Part model, mm, in its own coordinate system. A direction names the side the tool comes from. Round coordinates to 2 decimals unless told otherwise and drop trailing zeros. Order: outer loops, then holes, each group sorted by start corner. A loop starts at its lowest first (then second) coordinate and runs counter-clockwise, first axis right, second up. Notation, with made-up numbers: (-16, 84) -> (4, 84) arc R5 ccw to (4, 93) -> close; hole circle Ø2 at (51.5, -22). An arc over 180 degrees is marked (long way). Answer as a JSON object with one key per item and string values. Group by question number.
```python
from build123d import *

# Parameters (mm, degrees)
CUT_EXTRUDE1_DEPTH      = 10
CUT_EXTRUDE1_DEPTH_BACK = 10
SKETCH7_W               = 161.67088451347962
SKETCH7_H               = 99.40268669666085
SKETCH8_W               = 4.999999999999993
SKETCH8_H               = 94
CUT_EXTRUDE2_DEPTH      = 35
SKETCH9_R               = 7.5
SKETCH9_R_2             = 4.000000000000013
SKETCH9_R_3             = 4.000000000000005
CUT_EXTRUDE3_DEPTH      = 357.06460088023357
SKETCH10_R              = 4.000000000000005
CUT_EXTRUDE4_DEPTH      = 386.9080201291493
SKETCH11_W              = 141.9999999999999
SKETCH11_H              = 16
BOSS_EXTRUDE1_DEPTH     = 330
FILLET2_R               = 5
FILLET3_R               = 5
FILLET4_R               = 5
FILLET5_R               = 5
FILLET6_R               = 5
CUT_EXTRUDE5_DEPTH      = 389.0992141192763


with BuildPart() as part:
    # Sweep2: sweep along a path in Sketch4
    with BuildLine(Plane.XY) as sweep2_path:
        Line((-65, 350), (-64.99999999999994, 10.000000000000007))
        ThreePointArc((-64.99999999999994, 10.000000000000007), (-62.07106781186544, 2.928932188134527), (-54.99999999999996, 0))
        Line((-54.99999999999996, 0), (54.99999999999999, 0))
        ThreePointArc((54.99999999999999, 0), (62.071067811865476, 2.9289321881345227), (65, 10))
        Line((65, 10), (65, 350))
        Line((65, 350), (-65, 350))
    # Sketch6 → Sweep2 (sweep)
    with BuildSketch(Plane(origin=(0, 0, 0), x_dir=(0, 0, -1), z_dir=(1, 0, 0))):
        Polygon((45.00000000000006, 355.99999999999994), (-44.999999999999936, 355.99999999999994), (-44.999999999999936, 343.99999999999994), (45.000000000000064, 344), align=None)
    sweep(path=sweep2_path.line, transition=Transition.RIGHT)

    # Sketch7 → Cut-Extrude1 (cut, two sides: drawn at the far end of the back side and taken through both)
    with BuildSketch(Plane(origin=(0, 0, 0), x_dir=(1, 0, 0), z_dir=(0, 1, 0)).offset(-CUT_EXTRUDE1_DEPTH_BACK)):
        Rectangle(SKETCH7_W, SKETCH7_H)
    extrude(amount=CUT_EXTRUDE1_DEPTH + CUT_EXTRUDE1_DEPTH_BACK, mode=Mode.SUBTRACT)

    # Sketch8 → Cut-Extrude2 (cut)
    with BuildSketch(Plane(origin=(0, 0, 0), x_dir=(1, 0, 0), z_dir=(0, 1, 0))):
        with Locations((-65.5, 0.24224418482823395)):
            Rectangle(SKETCH8_W, SKETCH8_H)
        with Locations((65.5, 0.24224418482823395)):
            Rectangle(SKETCH8_W, SKETCH8_H)
    extrude(amount=CUT_EXTRUDE2_DEPTH, mode=Mode.SUBTRACT)

    # Sketch9 → Cut-Extrude3 (cut, through all)
    with BuildSketch(Plane(origin=(0, 355.99999999999994, 0), x_dir=(1, 0, 0), z_dir=(0, 1, 0))):
        with Locations(Location((0, 0, 0), (0, 0, 270))):
            Circle(SKETCH9_R)
        with Locations(Location((-42, 31.999999999999993, 0), (0, 0, 270))):
            Circle(SKETCH9_R_2)
        with Locations(Location((-42, -32.00000000000001, 0), (0, 0, 270))):
            Circle(SKETCH9_R_3)
        with Locations(Location((42, -31.999999999999954, 0), (0, 0, 90))):
            Circle(SKETCH9_R_3)
        with Locations(Location((42, 32, 0), (0, 0, 90))):
            Circle(SKETCH9_R_2)
    extrude(amount=-CUT_EXTRUDE3_DEPTH, mode=Mode.SUBTRACT)

    # Sketch10 → Cut-Extrude4 (cut, through all)
    with BuildSketch(Plane(origin=(70.99999999999996, 0, 0), x_dir=(0, 0, -1), z_dir=(1, 0, 0))):
        with Locations((-37.999999999999936, 17.000000000000014)):
            Circle(SKETCH10_R)
    extrude(amount=-CUT_EXTRUDE4_DEPTH, mode=Mode.SUBTRACT)

    # Sketch11 → Boss-Extrude1 (add)
    with BuildSketch(Plane(origin=(0, 355.99999999999994, 0), x_dir=(1, 0, 0), z_dir=(0, 1, 0))):
        with Locations((0, -52.999999999999936)):
            Rectangle(SKETCH11_W, SKETCH11_H)
    extrude(amount=-BOSS_EXTRUDE1_DEPTH)

    # Fillet2
    fillet2_edges = [part.edges().sort_by_distance(p)[0] for p in [
        (59.00000000000001, 177, -45.000000000000064),
    ]]
    fillet(fillet2_edges, radius=FILLET2_R)

    # Fillet3
    fillet3_edges = [part.edges().sort_by_distance(p)[0] for p in [
        (70.99999999999994, 182.99999999999997, -45.00000000000005),
    ]]
    fillet(fillet3_edges, radius=FILLET3_R)

    # Fillet4
    fillet4_edges = [part.edges().sort_by_distance(p)[0] for p in [
        (-59.00000000000001, 177, -45.000000000000064),
    ]]
    fillet(fillet4_edges, radius=FILLET4_R)

    # Fillet5
    fillet5_edges = [part.edges().sort_by_distance(p)[0] for p in [
        (-70.99999999999994, 182.99999999999997, -45.00000000000005),
    ]]
    fillet(fillet5_edges, radius=FILLET5_R)

    # Fillet6
    fillet6_edges = [part.edges().sort_by_distance(p)[0] for p in [
        (70.99999999999994, 355.99999999999994, 10.499999999999893),
        (69.53553390593268, 355.9999999999999, -43.535533905932894),
        (0, 355.99999999999994, -45.00000000000005),
        (0, 355.99999999999994, -45.00000000000005),
        (-69.53553390593268, 355.99999999999994, -43.535533905932795),
        (-70.99999999999994, 355.99999999999994, 10.499999999999936),
        (0, 355.99999999999994, 60.999999999999936),
        (-70.99999999999994, 190.99999999999994, 60.999999999999936),
        (70.99999999999994, 190.99999999999994, 60.999999999999936),
    ]]
    fillet(fillet6_edges, radius=FILLET6_R)

    # Sketch12 → Cut-Extrude5 (cut, through all)
    with BuildSketch(Plane.ZY.offset(70.9999999999999)):
        with BuildLine():
            Line((-19.99811023879916, 9.999999999999995), (-79.77303285275339, 10.000000000000018))
            Line((-79.77303285275339, 10.000000000000018), (-79.77303285275339, 406.4421165391139))
            Line((-79.77303285275339, 406.4421165391139), (-12.883579031367276, 360.2403098799698))
            ThreePointArc((-12.883579031367276, 360.2403098799698), (-23.51999666611846, 185.26395577223084), (-19.99811023879916, 9.999999999999995))
        make_face()
    extrude(amount=-CUT_EXTRUDE5_DEPTH, mode=Mode.SUBTRACT)


solid = part.part
```
Q1. Wall check: line 1 (X direction, y = 350, z = 32); line 2 (X direction, y = 28, z = -2); line 3 (X direction, y = 148, z = -1.5). Give the ranges that are in metal, low to high. Write a range as [from, to].
Q2. Band-saw the part on C-C (y = 17). Count the separate pieces of the cut face and the enclosed holes in it, plus the area to 3 significant figures.
Q3. Which spindle directions (+Z, -Z, +X, -X, +Y, -Y) get a long thin tool onto all of the face, cutting with end or side? Do faces 4 (the flat face through (-68, 22, 12)), 5 (the cylindrical face through (62.78, 222.418, -22.447)). Say none if no direction does.
Q4. Band-saw the part on D-D (x = 20). List the corners of the cut face in (y, z).
Q5. Band-saw the part on A-A (z = 0). List the corners of the cut face in (x, y).
Q6. Drop flat-ended pins along their axis: pin 1 Ø2 at (x, y) = (-15, 68.5) entering from -Z; pin 2 Ø5.5 at (x, z) = (64.5, 25) entering from -Y; pin 3 Ø18 at (x, z) = (-10.5, 13.5) entering from -Y; pin 4 Ø13 at (x, z) = (-8, 54.5) entering from -Y. Give the stop position or say it passes through.
Q7. Two-plate mould, pull along Z, no slides. Class faces 1 (the flat face through (-1, 191, 61)), 2 (the flat face through (-1, 344, 16)), 3 (the cylindrical face through (-69.48, 19.7, 40.95)): +Z half, -Z half, draft (parallel to the pull), parting line (faces both ways), or undercut.
Q8. Band-saw the part on B-B (x = 42). List the corners of the cut face in (y, z), plus the area to 3 significant figures.
Completed:
{
 "1": {"line 1": "[-71, -46], [-38, 38], [46, 71]", "line 2": "[-71, -68], [-63, -59], [59, 63], [68, 71]", "line 3": "[-71, -59], [59, 71]"},
 "2": {"separate pieces": "8", "enclosed holes": "0", "area": "804 mm2"},
 "3": {"face 4": "-Z, -Y", "face 5": "-Z, +X, -X"},
 "4": {"outline": "(26, 45) -> (344, 45) -> (344, -14.47) arc R2170 ccw to (356, -13.31) -> (356, 56) arc R5 ccw to (351, 61) -> (26, 61) -> close"},
 "5": {"outline": "(-71, 10) -> (-68, 10) -> (-68, 35) -> (-63, 35) -> (-63, 10) -> (-59, 10) -> (-59, 344) -> (-7.5, 344) -> (-7.5, 356) -> (-66, 356) arc R5 ccw to (-71, 351) -> close; (7.5, 344) -> (59, 344) -> (59, 10) -> (63, 10) -> (63, 35) -> (68, 35) -> (68, 10) -> (71, 10) -> (71, 351) arc R5 ccw to (66, 356) -> (7.5, 356) -> close"},
 "6": {"pin 1": "z = 45", "pin 2": "y = 10", "pin 3": "y = 344", "pin 4": "y = 26"},
 "7": {"face 1": "+Z half", "face 2": "draft", "face 3": "undercut"},
 "8": {"outline": "(26, 45) -> (344, 45) -> (344, 36) -> (356, 36) -> (356, 56) arc R5 ccw to (351, 61) -> (26, 61) -> close; (344, -14.47) arc R2170 ccw to (356, -13.31) -> (356, 28) -> (344, 28) -> close", "area": "5,890 mm2"}
}
